Can you work these out from the model? Positions are in its coordinate system, mm. Face numbers are marked on the shaded views. Coordinates: 2 decimals unless noted, no trailing zeros. Order: outer loops, then holes, each group sorted by start corner. A loop starts at its lowest first (then second) coordinate and runs counter-clockwise, first axis right, second up. Notation, with made-up numbers: (17, 82) -> (23, 82) arc R16 cw to (23, 87) -> close; hole circle Ø8 at (82.25, -13.75). An arc over 180 degrees is marked (long way). Answer in a Markdown table with one row per item.
```python
from build123d import *

# Parameters (mm, degrees)
BOSS_EXTRUDE1_DEPTH = 2


with BuildPart() as part:
    # Sketch1 → Boss-Extrude1 (new body)
    with BuildSketch(Plane(origin=(0, 0, 0), x_dir=(1, 0, 0), z_dir=(0, 1, 0))):
        with BuildLine():
            Line((35, 7.5), (26.5, 7.5))
            ThreePointArc((26.5, 7.5), (25, 6), (23.5, 7.5))
            Line((23.5, 7.5), (11.5, 7.5))
            ThreePointArc((11.5, 7.5), (10, 6), (8.5, 7.5))
            Line((8.5, 7.5), (0, 7.5))
            Line((0, 7.5), (0, 0))
            Line((0, 0), (35, 0))
            Line((35, 0), (35, 7.5))
        make_face()
        with BuildLine():
            ThreePointArc((23.5, 7.5), (25, 9), (26.5, 7.5))
            Line((26.5, 7.5), (35, 7.5))
            Line((35, 7.5), (35, 15))
            Line((35, 15), (0, 15))
            Line((0, 15), (0, 7.5))
            Line((0, 7.5), (8.5, 7.5))
            ThreePointArc((8.5, 7.5), (10, 9), (11.5, 7.5))
            Line((11.5, 7.5), (23.5, 7.5))
        make_face()
    extrude(amount=BOSS_EXTRUDE1_DEPTH)


solid = part.part
```
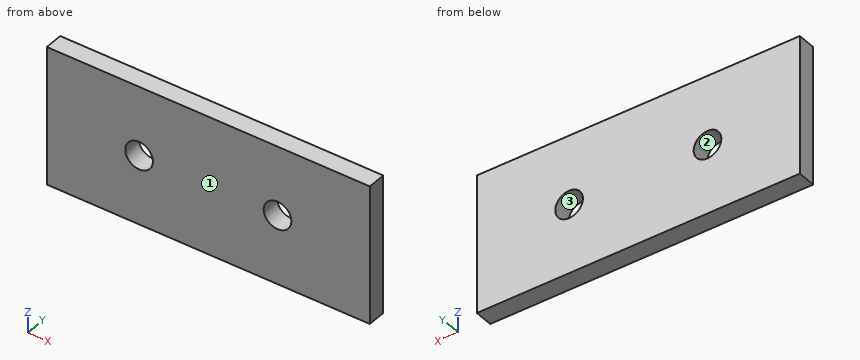
(1) We'd pull the mould along X, two halves only. Please class the marked faces 1, 2 and 3: +X half, -X half, draft (parallel to the pull), parting line (faces both ways), or undercut.
Response values:
| item | result |
|---|---|
| face 1 | draft |
| face 2 | undercut |
| face 3 | undercut |
(2) Suppose I cut it at B-B (x = 25). Please give me the cut outline in (y, z).
Response values:
| item | result |
|---|---|
| outline | (0, -15) -> (2, -15) -> (2, -9) -> (0, -9) -> close; (0, -6) -> (2, -6) -> (2, 0) -> (0, 0) -> close |
(3) Suppose I cut it at C-C (y = 1.55). Please give me the cut outline in (x, z), and give its area (3 significant figures).
Response values:
| item | result |
|---|---|
| outline | (0, -15) -> (35, -15) -> (35, 0) -> (0, 0) -> close; hole circle Ø3 at (10, -7.5); hole circle Ø3 at (25, -7.5) |
| area | 511 mm2 |
(4) Suppose I cut it at A-A (z = -7.5). Please give me the cut outline in (x, y), and give its area (3 significant figures).
Response values:
| item | result |
|---|---|
| outline | (0, 0) -> (8.5, 0) -> (8.5, 2) -> (0, 2) -> close; (11.5, 0) -> (23.5, 0) -> (23.5, 2) -> (11.5, 2) -> close; (26.5, 0) -> (35, 0) -> (35, 2) -> (26.5, 2) -> close |
| area | 58.0 mm2 |
(5) I need wall thicknesses on line 1 (X direction, y = 1, z = -7.5); line 2 (Z direction, x = 25, y = 0.7); line 3 (Z direction, x = 9.5, y = 1.55). Which ranges of each line are inside material? Lowest first, please. Write a range as [from, to].
Response values:
| item | result |
|---|---|
| line 1 | [0, 8.5], [11.5, 23.5], [26.5, 35] |
| line 2 | [-15, -9], [-6, 0] |
| line 3 | [-15, -8.91], [-6.09, 0] |
